```python
from build123d import *

# Parameters (mm, degrees)
SKETCH2_W                 = 8.4
SKETCH2_H                 = 10
BOSS_EXTRUDE1_DEPTH       = 11.3
SKETCH5_W                 = 8.4
SKETCH5_H                 = 1.5
CUT_EXTRUDE2_DEPTH        = 11.3
SKETCH7_W                 = 1.6
SKETCH7_H                 = 3.3
CUT_EXTRUDE4_DEPTH        = 8.4
SKETCH9_W                 = 8.4
SKETCH9_H                 = 1.7
CUT_EXTRUDE5_DEPTH        = 6.8
SKETCH12_W                = 6.8
SKETCH12_H                = 1.6
BOSS_EXTRUDE3_DEPTH       = 1.6
FILLET1_R                 = 1
M3X0_5_TAPPED_HOLE2_D     = 2.5
M3X0_5_TAPPED_HOLE2_DEPTH = 6.5
M3X0_5_TAPPED_HOLE2_TIP   = 0.751075774


with BuildPart() as part:
    # Sketch2 → Boss-Extrude1 (new body)
    with BuildSketch(Plane(origin=(0, 0, 0), x_dir=(1, 0, 0), z_dir=(0, 1, 0))):
        Rectangle(SKETCH2_W, SKETCH2_H)
    extrude(amount=BOSS_EXTRUDE1_DEPTH)

    # Sketch5 → Cut-Extrude2 (cut)
    with BuildSketch(Plane(origin=(4.2, 0, 0), x_dir=(0, 0, -1), z_dir=(1, 0, 0))):
        with Locations((0.8, 10.55)):
            Rectangle(SKETCH5_W, SKETCH5_H)
    extrude(amount=-CUT_EXTRUDE2_DEPTH, mode=Mode.SUBTRACT)

    # Sketch7 → Cut-Extrude4 (cut)
    with BuildSketch(Plane(origin=(0, 0, -5), x_dir=(-1, 0, 0), z_dir=(0, 0, -1))):
        with Locations((-3.4, 8.15)):
            Rectangle(SKETCH7_W, SKETCH7_H)
    extrude(amount=-CUT_EXTRUDE4_DEPTH, mode=Mode.SUBTRACT)

    # Sketch9 → Cut-Extrude5 (cut)
    with BuildSketch(Plane(origin=(2.6, 0, 0), x_dir=(0, 0, -1), z_dir=(1, 0, 0))):
        with Locations((0.8, 8.95)):
            Rectangle(SKETCH9_W, SKETCH9_H)
    extrude(amount=-CUT_EXTRUDE5_DEPTH, mode=Mode.SUBTRACT)

    # Sketch12 → Boss-Extrude3 (add)
    with BuildSketch(Plane(origin=(0, 0, 3.4), x_dir=(-1, 0, 0), z_dir=(0, 0, -1))):
        with Locations((0.8, 8.9)):
            Rectangle(SKETCH12_W, SKETCH12_H)
    extrude(amount=BOSS_EXTRUDE3_DEPTH)

    # Fillet1
    fillet1_edges = [part.edges().sort_by_distance(p)[0] for p in [
        (4.2, 3.25, -5),
        (0, 0, 5),
        (0, 0, -5),
        (4.2, 0, 0),
        (4.2, 5.65, 5),
    ]]
    fillet(fillet1_edges, radius=FILLET1_R)

    # M3x0.5 Tapped Hole2
    with Locations(Plane.ZY.offset(4.2)):
        with Locations((0, 5)):
            Hole(M3X0_5_TAPPED_HOLE2_D / 2, depth=M3X0_5_TAPPED_HOLE2_DEPTH)
            with Locations((0, 0, -(M3X0_5_TAPPED_HOLE2_DEPTH + M3X0_5_TAPPED_HOLE2_TIP / 2))):  # 118° drill point
                Cone(0, M3X0_5_TAPPED_HOLE2_D / 2, M3X0_5_TAPPED_HOLE2_TIP, mode=Mode.SUBTRACT)


solid = part.part
```
Design review of the part built by this model. Coordinates are the model's own, in mm. A direction names the side the tool comes from. Coordinates: 2 decimals unless noted, no trailing zeros. Write each loop counter-clockwise with the first axis right and the second up, starting at its lowest first coordinate (ties: lowest second). Pieces come first, ordered by that corner, then holes. Notation, with made-up numbers: M -25,53 L 22,53 A26 ccw 22,91 Z; hole C -30,-9 d11. An arc over 180 degrees is marked long. Answer as a JSON object with one key per item and string values.
Item 1: Add section A-A, the plane x = 1.25. Give the boundary of the cut face in (y, z), and give its area (3 significant figures).
Outcome:
{"outline": "M 0,-4 A1 ccw 1,-5 L 8.1,-5 L 8.1,1.8 L 9.7,1.8 L 9.7,3.4 L 11.3,3.4 L 11.3,5 L 1,5 A1 ccw 0,4 Z; hole C 5,0 d2.5", "area": "83.3 mm²"}
Item 2: Add section D-D, the plane z = -2. Give the boundary of the cut face in (x, y).
Outcome:
{"outline": "M -4.2,0 L 3.2,0 A1 ccw 4.2,1 L 4.2,6.5 L 2.6,6.5 L 2.6,8.1 L -4.2,8.1 Z"}
Item 3: Insertion check: pin 1 Ø1.5 at (x, y) = (-1, 9.5) entering from -Z; pin 2 Ø2.5 at (y, z) = (9, -1.5) entering from +X; pin 3 Ø0.5 at (x, z) = (-2.5, 3) entering from +Y. Each pin has a flat end and moves straight along its axis. Give the tip position at first contact, or say it passes through.
Outcome:
{"pin 1": "z = 1.8", "pin 2": "x = 2.6", "pin 3": "y = 9.7"}
Item 4: Add section B-B, the plane z = 2.25. Give the boundary of the cut face in (x, y), and give its area (3 significant figures).
Outcome:
{"outline": "M -4.2,0 L 3.2,0 A1 ccw 4.2,1 L 4.2,6.5 L 2.6,6.5 L 2.6,9.7 L -4.2,9.7 Z", "area": "76.1 mm²"}
Item 5: Draft analysis for pull direction Z (two halves, no side actions). For faces 1 (the flat face through (-1, 9.7, 3)), 2 (the flat face through (-1, 9, 1.8)), 3 (the conical face through (2.92, 5.18, 0.12)), state which applies: pulls with the +Z half, pulls with the -Z half, needs draft (parallel to the pull), parting line crosses it, or undercut.
Outcome:
{"face 1": "needs draft", "face 2": "pulls with the -Z half", "face 3": "undercut"}
Item 6: Add section C-C, the plane y = 10.75. Give the boundary of the cut face in (x, z).
Outcome:
{"outline": "M -4.2,3.4 L 4.2,3.4 L 4.2,4 A1 ccw 3.2,5 L -4.2,5 Z"}
Item 7: Wall thickness on probe 1 along Y at (x, z) = (-1.75, 0); probe 2 along Z at (x, y) = (0.25, 5); probe 3 along Y at (x, z) = (2, -1.75): over which ranges is each line inside the solid? List them lowest first.
Outcome:
{"probe 1": "0 to 3.75, 6.25 to 8.1", "probe 2": "-5 to -1.25, 1.25 to 5", "probe 3": "0 to 8.1"}
Item 8: Machinability: for faces 4 (the cylindrical face through (3.915, 6.222, 4.699)), 5 (the flat face through (-1, 8.1, -2)), 6 (the flat face through (3, 6.5, -1)), 7 (the cylindrical face through (-0.9, 3.78, 0.27)), 8 (the flat face through (-4.2, 4, 1)), which of the approach directions +Z, -Z, +X, -X, +Y, -Y give a long, thin tool a straight path to every point of the face, cutting with its end or side? Answer none if there is none.
Outcome:
{"face 4": "+Z, +X, +Y, -Y", "face 5": "-Z, +X, -X, +Y", "face 6": "-Z, +X, +Y", "face 7": "-X", "face 8": "+Z, -Z, -X, +Y, -Y"}
